from build123d import *

# Parameters (mm, degrees)
BOSS_EXTRUDE1_DEPTH = 1.5


with BuildPart() as part:
    # Sketch1 → Revolve1 (revolve)
    with BuildSketch(Plane.XY):
        Polygon((0, 0), (1.9, 0), (1.9, 13), (2.825, 13), (2.825, 14.5), (0, 14.5), align=None)
    revolve(axis=Axis((0, 0, 0), (0, 1, 0)))

    # Sketch2 → Boss-Extrude1 (add, symmetric)
    with BuildSketch(Plane.XY):
        with BuildLine():
            Line((-2.325, 14.5), (-2.325, 21.45))
            ThreePointArc((-2.325, 21.45), (-1.314518395, 23.889518395), (1.125, 24.9))
            Line((1.125, 24.9), (1.225, 24.9))
            ThreePointArc((1.225, 24.9), (3.664518395, 23.889518395), (4.675, 21.45))
            Line((4.675, 21.45), (4.675, 15.5))
            Line((4.675, 15.5), (2.575, 15))
            Line((2.575, 15), (2.575, 14.5))
            Line((2.575, 14.5), (-2.325, 14.5))
        make_face()
    extrude(amount=BOSS_EXTRUDE1_DEPTH, both=True)


solid = part.part
For this review, take the finished solid that the model builds, in its own axes (mm). A direction names the side the tool comes from. Give positions to 0.01 mm unless a question says otherwise; leave off trailing zeros. Order: outer loops, then holes, each group sorted by start corner. A loop starts at its lowest first (then second) coordinate and runs counter-clockwise, first axis right, second up. Notation, with made-up numbers: M 65.25,7.25 L 74.25,7.25 A21 ccw 74.25,45.25 Z; hole C -40,78.25 d2. An arc over 180 degrees is marked long. Answer in a Markdown table with one row per item. Add a question column.
(1) Consider section C-C on y = 18.75. State the section outline as (x, z) points (3 decimals).
(2) Consider section A-A on z = 0. State the section outline as (x, y) points (3 decimals), and give its area (3 significant figures).
(3) Consider section D-D on x = -1.25. State the section outline as (y, z) points, and give its area (3 significant figures).
(4) Wall thickness on probe 1 along Z at (x, y) = (-1.5, 22.25); probe 2 along Y at (x, z) = (-1.5, 1.55); probe 3 along X at (y, z) = (18.75, 0.95) (3 decimals): over which ranges is each line inside the solid? List them lowest first. Write a range as [from, to].
(5) For pin 1 (1 mm diameter, centred on x = 0.5, y = 20.5, fed in from +Z); pin 2 (0.9 mm diameter, centred on y = 16.5, z = 0.5, fed in from -X) (3 decimals), all flat-tipped, find the tip position at first contact; note any pin that passes through.
(6) Consider section B-B on x = 0.5. State the section outline as (y, z) points.
(7) For faces 1 (the face through (1, 20, -1.5)), 2 (the face through (1, 20, 1.5)), 3 (the face through (-2.325, 18, 0)), 4 (the face through (-1.9, 6.59, -0.08)), list the 3-axis set-ups (+Z, -Z, +X, -X, +Y, -Y) from which the entire face can be reached by the end or side of a thin tool; tool diameter is ignored.
Evaluation:
| question | item | result |
|---|---|---|
| 1 | outline | M -2.325,-1.5 L 4.675,-1.5 L 4.675,1.5 L -2.325,1.5 Z |
| 2 | outline | M -2.825,13 L -1.9,13 L -1.9,0 L 1.9,0 L 1.9,13 L 2.825,13 L 2.825,14.5 L 2.575,14.5 L 2.575,15 L 4.675,15.5 L 4.675,21.45 A3.45 ccw 1.225,24.9 L 1.125,24.9 A3.45 ccw -2.325,21.45 L -2.325,14.5 L -2.825,14.5 Z |
| 2 | area | 124 mm^2 |
| 3 | outline | M 0,-1.43 L 13,-1.43 L 13,-2.53 L 14.5,-2.53 L 14.5,-1.5 L 23.95,-1.5 L 23.95,1.5 L 14.5,1.5 L 14.5,2.53 L 13,2.53 L 13,1.43 L 0,1.43 Z |
| 3 | area | 73.2 mm^2 |
| 4 | probe 1 | z = [-1.5, 1.5] |
| 4 | probe 2 | y = [13, 14.5] |
| 4 | probe 3 | x = [-2.325, 4.675] |
| 5 | pin 1 | stops at z = 1.5 |
| 5 | pin 2 | stops at x = -2.325 |
| 6 | outline | M 0,-1.83 L 13,-1.83 L 13,-2.78 L 14.5,-2.78 L 14.5,-1.5 L 24.84,-1.5 L 24.84,1.5 L 14.5,1.5 L 14.5,2.78 L 13,2.78 L 13,1.83 L 0,1.83 Z |
| 7 | face 1 | -Z, +X, -X, +Y |
| 7 | face 2 | +Z, +X, -X, +Y |
| 7 | face 3 | +Z, -Z, -X, +Y |
| 7 | face 4 | -Y |
